```python
from build123d import *

# Parameters (mm, degrees)
SKETCH_1_W               = 67
SKETCH_1_H               = 39
EXTRUDE_1_DEPTH          = 2
SKETCH_2_R               = 2
CUT_EXTRUDE_1_DEPTH      = 2
MIRROR_2_COPY_1_SKETCH_R = 2
MIRROR_2_COPY_1_DEPTH    = 2
SKETCH_3_W               = 8
SKETCH_3_H               = 10
EXTRUDE_2_DEPTH          = 10
CUT_EXTRUDE_2_DEPTH      = 10
SKETCH_5_R               = 1.5
CUT_EXTRUDE_3_DEPTH      = 8
SKETCH_6_W               = 10
SKETCH_6_H               = 5
EXTRUDE_3_DEPTH          = 10
SKETCH_10_W              = 23
SKETCH_10_H              = 14
EXTRUDE_4_DEPTH          = 7.5


with BuildPart() as part:
    # 草图1 → 凸台-拉伸1 (new body)
    with BuildSketch(Plane.XY):
        Rectangle(SKETCH_1_W, SKETCH_1_H)
    extrude(amount=EXTRUDE_1_DEPTH)

    # 草图2 → 切除-拉伸1 (cut)
    with BuildSketch(Plane.XY.offset(2)):
        with Locations((-30.5, 16.5)):
            Circle(SKETCH_2_R)
    cut_extrude_1 = extrude(amount=-CUT_EXTRUDE_1_DEPTH, mode=Mode.SUBTRACT)

    # 镜向1: 切除-拉伸1 across plane
    add(cut_extrude_1.mirror(Plane(origin=(0, 0, 0), x_dir=(0, 0, 1), z_dir=(1, 0, 0))), mode=Mode.SUBTRACT)

    # 镜向2: 切除-拉伸1 across plane
    add(cut_extrude_1.mirror(Plane.ZX), mode=Mode.SUBTRACT)

    # 镜向2 copy 1 sketch → 镜向2 copy 1 (cut)
    with BuildSketch(Plane(origin=(0, 0, 2), x_dir=(-1, 0, 0), z_dir=(0, 0, 1))):
        with Locations((-30.5, 16.5)):
            Circle(MIRROR_2_COPY_1_SKETCH_R)
    extrude(amount=-MIRROR_2_COPY_1_DEPTH, mode=Mode.SUBTRACT)

    # 草图3 → 凸台-拉伸2 (add)
    with BuildSketch(Plane(origin=(0, 0, 0), x_dir=(-1, 0, 0), z_dir=(0, 0, -1))):
        with Locations((-29.5, 0)):
            Rectangle(SKETCH_3_W, SKETCH_3_H)
    extrude_2 = extrude(amount=EXTRUDE_2_DEPTH)

    # 草图4 → 切除-拉伸2 (cut)
    with BuildSketch(Plane.XZ.offset(5)):
        Polygon((32.5, -10), (33.5, -6), (33.5, -10), align=None)
        Polygon((25.5, -10), (25.5, -6), (26.5, -10), align=None)
    cut_extrude_2 = extrude(amount=-CUT_EXTRUDE_2_DEPTH, mode=Mode.SUBTRACT)

    # 草图5 → 切除-拉伸3 (cut)
    with BuildSketch(Plane(origin=(0, 0, -10), x_dir=(-1, 0, 0), z_dir=(0, 0, -1))):
        with Locations((-29.5, 2)):
            Circle(SKETCH_5_R)
        with Locations((-29.5, -2)):
            Circle(SKETCH_5_R)
    cut_extrude_3 = extrude(amount=-CUT_EXTRUDE_3_DEPTH, mode=Mode.SUBTRACT)

    # 镜向3: 凸台-拉伸2, 切除-拉伸2, 切除-拉伸3 across plane
    add(extrude_2.mirror(Plane(origin=(0, 0, 0), x_dir=(0, 0, 1), z_dir=(1, 0, 0))))
    add(cut_extrude_2.mirror(Plane(origin=(0, 0, 0), x_dir=(0, 0, 1), z_dir=(1, 0, 0))), mode=Mode.SUBTRACT)
    add(cut_extrude_3.mirror(Plane(origin=(0, 0, 0), x_dir=(0, 0, 1), z_dir=(1, 0, 0))), mode=Mode.SUBTRACT)

    # 草图6 → 凸台-拉伸3 (add)
    with BuildSketch(Plane(origin=(0, 0, 0), x_dir=(-1, 0, 0), z_dir=(0, 0, -1))):
        with Locations((0, 17)):
            Rectangle(SKETCH_6_W, SKETCH_6_H)
    extrude(amount=EXTRUDE_3_DEPTH)

    # 草图10 → 凸台-拉伸4 (add)
    with BuildSketch(Plane(origin=(0, 0, 0), x_dir=(-1, 0, 0), z_dir=(0, 0, -1))):
        with Locations((0, -12.5)):
            Rectangle(SKETCH_10_W, SKETCH_10_H)
    extrude(amount=EXTRUDE_4_DEPTH)


solid = part.part
```
Source: CAD feature listing. Evaluate the final solid. Frame: model axes, mm. A direction names the side the tool comes from. Coordinates: 2 decimals unless noted, no trailing zeros. Order: outer loops, then holes, each group sorted by start corner. A loop starts at its lowest first (then second) coordinate and runs counter-clockwise, first axis right, second up. Notation, with made-up numbers: (38.5, 72) - (78.5, 72) arc R26 cw to (78.5, 95) - close; hole circle Ø9 at (-31, 20.25). An arc over 180 degrees is marked (long way). One line per item, written item: value.
1) Cut plane B-B on z = -3. Output: boundary loops of the cut face in (x, y).
Computed values:
outline: (-33.5, -5) - (-25.5, -5) - (-25.5, 5) - (-33.5, 5) - close; (-11.5, -19.5) - (11.5, -19.5) - (11.5, -5.5) - (-11.5, -5.5) - close; (-5, 14.5) - (5, 14.5) - (5, 19.5) - (-5, 19.5) - close; (25.5, -5) - (33.5, -5) - (33.5, 5) - (25.5, 5) - close; hole circle Ø3 at (-29.5, -2); hole circle Ø3 at (-29.5, 2); hole circle Ø3 at (29.5, -2); hole circle Ø3 at (29.5, 2)
2) Ray query, line 1 (Y direction, x = -29.5, z = -5.25); line 2 (X direction, y = -16.5, z = 1.45); line 3 (Y direction, x = 30.5, z = 1.05). Return the intervals inside material, ascending. Write a range as [from, to].
Computed values:
line 1: y = [-5, -3.5], [-0.5, 0.5], [3.5, 5]
line 2: x = [-33.5, -32.5], [-28.5, 28.5], [32.5, 33.5]
line 3: y = [-19.5, -18.5], [-14.5, 14.5], [18.5, 19.5]
3) Mould query, pull axis X, two halves, no side actions, for faces 1 (the face through (-33.5, 0, -1)), 2 (the face through (-28.592, 17.101, 1.014)), 3 (the face through (33.5, 0, -1)), 4 (the face through (0, -12, -7.5)). Classes: released by +X, released by -X, zero draft, split by the parting line, or undercut.
Computed values:
face 1: released by -X
face 2: undercut
face 3: released by +X
face 4: zero draft
4) Cut plane A-A on y = 16.5. Output: boundary loops of the cut face in (x, z), plus the area to 3 significant figures.
Computed values:
outline: (-33.5, 0) - (-32.5, 0) - (-32.5, 2) - (-33.5, 2) - close; (-28.5, 0) - (-5, 0) - (-5, -10) - (5, -10) - (5, 0) - (28.5, 0) - (28.5, 2) - (-28.5, 2) - close; (32.5, 0) - (33.5, 0) - (33.5, 2) - (32.5, 2) - close
area: 218 mm^2
5) Cut plane D-D on y = -2. Output: boundary loops of the cut face in (x, z).
Computed values:
outline: (-33.5, -6) - (-32.5, -10) - (-31, -10) - (-31, -2) - (-28, -2) - (-28, -10) - (-26.5, -10) - (-25.5, -6) - (-25.5, 0) - (25.5, 0) - (25.5, -6) - (26.5, -10) - (28, -10) - (28, -2) - (31, -2) - (31, -10) - (32.5, -10) - (33.5, -6) - (33.5, 2) - (-33.5, 2) - close
6) Reachability of faces 5 (the face through (11.5, -13, -4)), 6 (the face through (30, -5, -5)), 7 (the face through (30, 5, -5)), 8 (the face through (26, 0, -8)) from +Z, -Z, +X, -X, +Y, -Y: full face, straight path, thin tool, end or side. Return the list, or none.
Computed values:
face 5: -Z, +X, +Y, -Y
face 6: -Z, +X, -X, -Y
face 7: -Z, +X, -X, +Y
face 8: -Z, +Y, -Y
7) Cut plane C-C on x = -29.5. Output: boundary loops of the cut face in (y, z), plus the area to 3 significant figures.
Computed values:
outline: (-19.5, 0) - (-18.23, 0) - (-18.23, 2) - (-19.5, 2) - close; (-14.77, 0) - (-5, 0) - (-5, -10) - (-3.5, -10) - (-3.5, -2) - (-0.5, -2) - (-0.5, -10) - (0.5, -10) - (0.5, -2) - (3.5, -2) - (3.5, -10) - (5, -10) - (5, 0) - (14.77, 0) - (14.77, 2) - (-14.77, 2) - close; (18.23, 0) - (19.5, 0) - (19.5, 2) - (18.23, 2) - close
area: 116 mm^2
8) Contact query for flat-ended pins moving along their axis: pin 1 (2.5 mm diameter, centred on x = 31.5, z = -6.5, fed in from -Y); pin 2 (5 mm diameter, centred on x = 26, z = -7.5, fed in from +Y); pin 3 (12 mm diameter, centred on x = -4.5, y = -14.5, fed in from -Z). Output: stop coordinate, or through.
Computed values:
pin 1: stops at y = -5
pin 2: stops at y = 5
pin 3: stops at z = -7.5
